Work out the finished part from the listing and answer in its coordinate system (mm). Face numbers are marked on the shaded views. A direction names the side the tool comes from. Round coordinates to 2 decimals unless told otherwise and drop trailing zeros. Loops run counter-clockwise (first coordinate to the right, second up) from the corner with the lowest first, then second, coordinate; pieces in that order, holes last. Notation, with made-up numbers: (68, 12) - (113, 12) arc R18 ccw to (113, 37) - close; hole circle Ø4 at (35.5, 37). An arc over 180 degrees is marked (long way). Return JSON: item names as keys, results as strings.
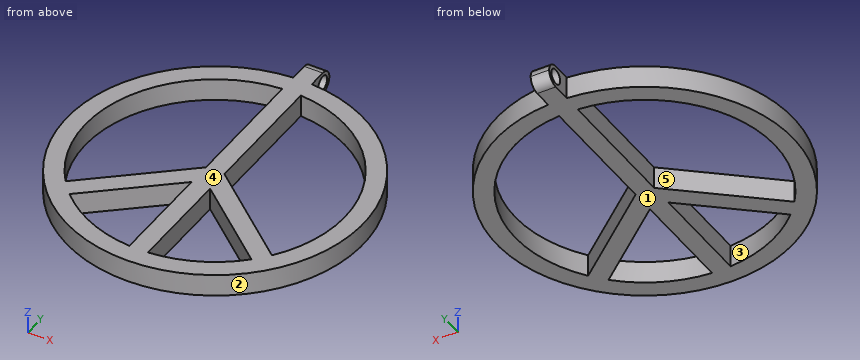
from build123d import *

# Parameters (mm, degrees)
F1_DEPTH = 7.62
F2_R     = 2.54
F3_DEPTH = 25.4


with BuildPart() as f1:
    # F0 (on Top) → F1 (new body)
    with BuildSketch(Plane.XY):
        with BuildLine():
            Line((-3.175, 60.860684), (-3.175, 50.700684))
            ThreePointArc((-3.175, 50.700684), (0, -50.8), (3.175, 50.700684))
            Line((3.175, 50.700684), (3.175, 60.860684))
            Line((3.175, 60.860684), (-3.175, 60.860684))
        make_face()
        with BuildLine():
            Line((-31.192057, -31.667934), (-3.175, -8.272762))
            Line((-3.175, -8.272762), (-3.175, -44.336462))
            ThreePointArc((-3.175, -44.336462), (-18.313835, -40.501925), (-31.192057, -31.667934))
        make_face(mode=Mode.SUBTRACT)
        with BuildLine():
            Line((3.175, -44.336462), (3.175, -8.272762))
            Line((3.175, -8.272762), (31.192057, -31.667934))
            ThreePointArc((31.192057, -31.667934), (18.313835, -40.501925), (3.175, -44.336462))
        make_face(mode=Mode.SUBTRACT)
        with BuildLine():
            ThreePointArc((-35.38748, -26.89849), (-40.501491, 18.314794), (-3.175, 44.336462))
            Line((-3.175, 44.336462), (-3.175, 0))
            Line((-3.175, 0), (-35.38748, -26.89849))
        make_face(mode=Mode.SUBTRACT)
        with BuildLine():
            Line((3.175, 0), (3.175, 44.336462))
            ThreePointArc((3.175, 44.336462), (40.501491, 18.314794), (35.38748, -26.89849))
            Line((35.38748, -26.89849), (3.175, 0))
        make_face(mode=Mode.SUBTRACT)
    extrude(amount=F1_DEPTH)

    # F2 (on face) → F3 (cut)
    with BuildSketch(Plane(origin=(-3.175, 0, 0), x_dir=(0, -1, 0), z_dir=(-1, 0, 0))):
        with Locations((-57.050684, 3.81)):
            Circle(F2_R)
        with BuildLine():
            ThreePointArc((-60.860684, 3.81), (-59.744761, 6.504077), (-57.050684, 7.62))
            Line((-57.050684, 7.62), (-60.860684, 7.62))
            Line((-60.860684, 7.62), (-60.860684, 3.81))
        make_face()
        with BuildLine():
            Line((-60.860684, 0), (-57.050684, 0))
            ThreePointArc((-57.050684, 0), (-59.744761, 1.115923), (-60.860684, 3.81))
            Line((-60.860684, 3.81), (-60.860684, 0))
        make_face()
    extrude(amount=-F3_DEPTH, mode=Mode.SUBTRACT)


solid = f1.part
1) Flat-ended cylindrical pins translate along their axes: pin 1 (4 mm diameter, centred on y = -22, z = 2, fed in from +X); pin 2 (4 mm diameter, centred on y = 56, z = 5.5, fed in from -X) (3 decimals); pin 3 (2.5 mm diameter, centred on y = 53.5, z = 5.5, fed in from +X) (3 decimals); pin 4 (4.5 mm diameter, centred on y = 57.05, z = 3.81, fed in from -X). Find the tip coordinate at first contact, or state that the pin passes through.
Verdict:
{"pin 1": "stops at x = 46.7", "pin 2": "stops at x = -3.175", "pin 3": "stops at x = 3.175", "pin 4": "passes through"}
2) Section B-B (x = -17.5) is taken. Give the vertices of the cut face in (y, z).
Verdict:
{"outline": "(-47.69, 0) - (-40.86, 0) - (-40.86, 7.62) - (-47.69, 7.62) - close; (-20.23, 0) - (-11.96, 0) - (-11.96, 7.62) - (-20.23, 7.62) - close; (40.86, 0) - (47.69, 0) - (47.69, 7.62) - (40.86, 7.62) - close"}
3) Section A-A (z = 5) is taken. Give the vertices of the cut face in (x, y) (3 decimals), and give its area (3 significant figures).
Verdict:
{"outline": "(-3.175, 50.701) arc R50.8 ccw (long way) to (3.175, 50.701) - (3.175, 54.807) - (-3.175, 54.807) - close; (-3.175, 59.295) - (3.175, 59.295) - (3.175, 60.67) - (-3.175, 60.67) - close; hole (-35.387, -26.898) - (-3.175, 0) - (-3.175, 44.336) arc R44.45 ccw to start; hole (-31.192, -31.668) arc R44.45 ccw to (-3.175, -44.336) - (-3.175, -8.273) - close; hole (3.175, -44.336) arc R44.45 ccw to (31.192, -31.668) - (3.175, -8.273) - close; hole (3.175, 0) - (35.387, -26.898) arc R44.45 ccw to (3.175, 44.336) - close", "area": "3,000 mm2"}
4) A tool of negligible diameter and unlimited length cuts with its end or side. For the marked faces 4 and 5, from which of +Z, -Z, +X, -X, +Y, -Y can it reach the whole face along a straight path? Write none if from no direction.
Verdict:
{"face 4": "+Z, +X, -X, +Y, -Y", "face 5": "+Z, -Z"}
5) Section D-D (x = 0) is taken. Give the vertices of the cut face in (y, z).
Verdict:
{"outline": "(-50.8, 0) - (57.05, 0) arc R3.81 ccw to (60.86, 3.81) arc R3.81 ccw to (57.05, 7.62) - (-50.8, 7.62) - close; hole circle Ø5.08 at (57.05, 3.81)"}
6) Section C-C (y = -11.5) is taken. Give the vertices of the cut face in (x, z) (3 decimals).
Verdict:
{"outline": "(-49.481, 0) - (-42.937, 0) - (-42.937, 7.62) - (-49.481, 7.62) - close; (-16.947, 0) - (-7.04, 0) - (-7.04, 7.62) - (-16.947, 7.62) - close; (-3.175, 0) - (3.175, 0) - (3.175, 7.62) - (-3.175, 7.62) - close; (7.04, 0) - (16.947, 0) - (16.947, 7.62) - (7.04, 7.62) - close; (42.937, 0) - (49.481, 0) - (49.481, 7.62) - (42.937, 7.62) - close"}
7) Determine the mould class of the marked faces 1, 2 and 3 for opening direction Y: pulls with the +Y half, pulls with the -Y half, needs draft (parallel to the pull), parting line crosses it, or undercut.
Verdict:
{"face 1": "needs draft", "face 2": "parting line crosses it", "face 3": "undercut"}
8) Find the intervals of material crossed by L1, parallel to Y at x = 20, z = 4.5; L2, parallel to X at y = -38, z = 1 (3 decimals); L3, parallel to X at y = 19, z = 3.25 (3 decimals), in increasing order.
Verdict:
{"L1": "y = -46.7 to -39.7, -22.32 to -14.05, 39.7 to 46.7", "L2": "x = -33.714 to -23.061, -3.175 to 3.175, 23.061 to 33.714", "L3": "x = -47.113 to -40.185, -3.175 to 3.175, 40.185 to 47.113"}
